Design review of the part built by this model. Coordinates are the model's own, in mm. Round coordinates to 2 decimals unless told otherwise and drop trailing zeros. Order: outer loops, then holes, each group sorted by start corner. A loop starts at its lowest first (then second) coordinate and runs counter-clockwise, first axis right, second up. Notation, with made-up numbers: (-3, 65) - (25, 65) arc R15 cw to (25, 82) - close; hole circle Ø9 at (45.25, -3.5). An arc over 180 degrees is marked (long way). Write item = value, one per line.
from build123d import *

# Parameters (mm, degrees)
SKETCH_1_W          = 98
SKETCH_1_H          = 200
EXTRUDE_1_DEPTH     = 42
SKETCH_2_R          = 1.5
CUT_EXTRUDE_3_DEPTH = 5
SKETCH_3_W          = 96.5
SKETCH_3_H          = 10
CUT_EXTRUDE_4_DEPTH = 34
SKETCH_4_W          = 68
SKETCH_4_H          = 13
EXTRUDE_2_DEPTH     = 13


with BuildPart() as part:
    # Эскиз1 → Бобышка-Вытянуть1 (new body)
    with BuildSketch(Plane.XY):
        with Locations((30.809352232, -67.603045404)):
            Rectangle(SKETCH_1_W, SKETCH_1_H)
    extrude(amount=EXTRUDE_1_DEPTH)

    # Эскиз2 → Вырез-Вытянуть3 (cut)
    with BuildSketch(Plane.XY):
        with Locations((-9.190647768, -30.103045404)):
            Circle(SKETCH_2_R)
        with Locations((70.809352232, -30.103045404)):
            Circle(SKETCH_2_R)
        with Locations((-9.190647768, -150.103045404)):
            Circle(SKETCH_2_R)
        with Locations((70.809352232, -150.103045404)):
            Circle(SKETCH_2_R)
    extrude(amount=CUT_EXTRUDE_3_DEPTH, mode=Mode.SUBTRACT)

    # Эскиз3 → Вырез-Вытянуть4 (cut)
    with BuildSketch(Plane.XY.offset(42)):
        with Locations((31.559352232, 27.396954596)):
            Rectangle(SKETCH_3_W, SKETCH_3_H)
    extrude(amount=-CUT_EXTRUDE_4_DEPTH, mode=Mode.SUBTRACT)

    # Эскиз4 → Бобышка-Вытянуть2 (add)
    with BuildSketch(Plane(origin=(0, 22.396954596, 0), x_dir=(1, 0, 0), z_dir=(0, 1, 0))):
        with Locations((34.309352232, -14.5)):
            Rectangle(SKETCH_4_W, SKETCH_4_H)
    extrude(amount=EXTRUDE_2_DEPTH)


solid = part.part
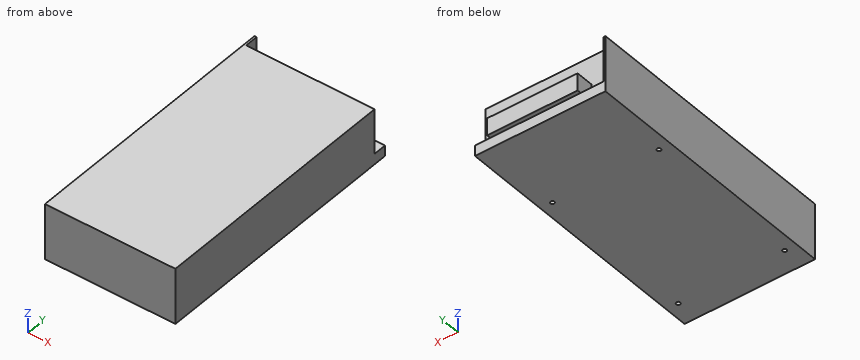
Item 1: Take a section at C-C, the plane z = 34. State the section outline as (x, y) points.
Data:
outline = (-18.19, -167.6) - (79.81, -167.6) - (79.81, 22.4) - (-16.69, 22.4) - (-16.69, 32.4) - (-18.19, 32.4) - close
Item 2: Take a section at A-A, the plane z = 18. State the section outline as (x, y) points, and give its area (3 significant figures).
Data:
outline = (-18.19, -167.6) - (79.81, -167.6) - (79.81, 22.4) - (68.31, 22.4) - (68.31, 35.4) - (0.31, 35.4) - (0.31, 22.4) - (-16.69, 22.4) - (-16.69, 32.4) - (-18.19, 32.4) - close
area = 19,500 mm2
Item 3: Take a section at D-D, the plane x = -5.5. State the section outline as (y, z) points.
Data:
outline = (-167.6, 0) - (32.4, 0) - (32.4, 8) - (22.4, 8) - (22.4, 42) - (-167.6, 42) - close
Item 4: For line 1 along Y through (x, z) = (-8.5, 2); line 2 along Y through (x, z) = (-5.5, 34.5); line 3 along Y through (x, z) = (-10, 5.5), list the stretches that pass through material, from the lowest coordinate up. Write a range as [from, to].
Data:
line_1 = [-167.6, -151.43], [-148.77, -31.43], [-28.77, 32.4]
line_2 = [-167.6, 22.4]
line_3 = [-167.6, 32.4]
Item 5: Insertion check: P1, Ø1.5, axis at x = -9.5, y = -29.5, coming from the -Z side; P2, Ø5, axis at x = -11.5, y = 28.5, coming from the +Z side; P3, Ø0.9, axis at x = 19.5, y = 34, coming from the -Z side. Each pin has a flat end and moves straight along its axis. Give the tip position at first contact, or say it passes through.
Data:
P1 = 5
P2 = 8
P3 = 8
Item 6: Take a section at B-B, the plane x = 59.5. State the section outline as (y, z) points.
Data:
outline = (-167.6, 0) - (32.4, 0) - (32.4, 8) - (35.4, 8) - (35.4, 21) - (22.4, 21) - (22.4, 42) - (-167.6, 42) - close
